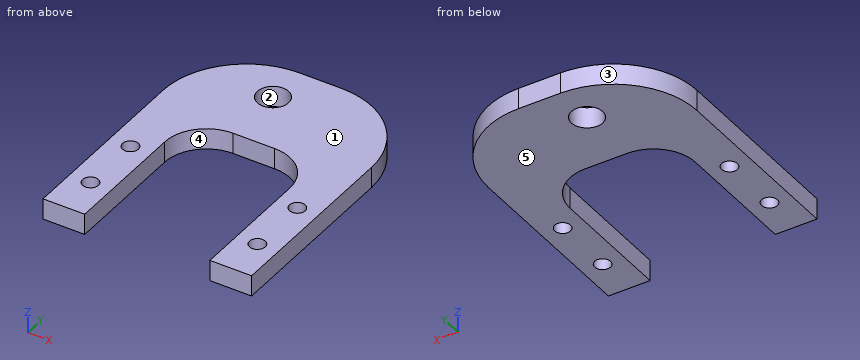
from build123d import *

# Parameters (mm, degrees)
BOSS_EXTRUDE1_DEPTH = 6.35
CUT_EXTRUDE1_REACH  = 8.35
SKETCH2_R           = 2.413
CUT_EXTRUDE2_REACH  = 8.35
SKETCH3_R           = 4.7625
FILLET1_R           = 12.7
FILLET2_R           = 25.4


with BuildPart() as part:
    # Sketch1 → Boss-Extrude1 (new body)
    with BuildSketch(Plane.XY):
        Polygon((0, 0), (12.7, 0), (12.7, 50.8), (50.8, 50.8), (50.8, 0), (63.5, 0), (63.5, 82.55), (0, 82.55), align=None)
    extrude(amount=BOSS_EXTRUDE1_DEPTH)

    # Sketch2 → Cut-Extrude1 (cut, up to next)
    with BuildSketch(Plane.XY.offset(6.35), mode=Mode.PRIVATE) as cut_extrude1_sk1:
        with Locations((6.35, 12.7)):
            Circle(SKETCH2_R)
    cut_extrude1_tool1 = extrude(cut_extrude1_sk1.sketch, amount=-CUT_EXTRUDE1_REACH, mode=Mode.PRIVATE) & part.part
    add(cut_extrude1_tool1.solids().sort_by_distance((6.35, 12.7, 6.35))[0], mode=Mode.SUBTRACT)
    # Sketch2 → Cut-Extrude1 (cut, up to next)
    with BuildSketch(Plane.XY.offset(6.35), mode=Mode.PRIVATE) as cut_extrude1_sk2:
        with Locations((6.35, 31.75)):
            Circle(SKETCH2_R)
    cut_extrude1_tool2 = extrude(cut_extrude1_sk2.sketch, amount=-CUT_EXTRUDE1_REACH, mode=Mode.PRIVATE) & part.part
    add(cut_extrude1_tool2.solids().sort_by_distance((6.35, 31.75, 6.35))[0], mode=Mode.SUBTRACT)
    # Sketch2 → Cut-Extrude1 (cut, up to next)
    with BuildSketch(Plane.XY.offset(6.35), mode=Mode.PRIVATE) as cut_extrude1_sk3:
        with Locations((57.15, 12.7)):
            Circle(SKETCH2_R)
    cut_extrude1_tool3 = extrude(cut_extrude1_sk3.sketch, amount=-CUT_EXTRUDE1_REACH, mode=Mode.PRIVATE) & part.part
    add(cut_extrude1_tool3.solids().sort_by_distance((57.15, 12.7, 6.35))[0], mode=Mode.SUBTRACT)
    # Sketch2 → Cut-Extrude1 (cut, up to next)
    with BuildSketch(Plane.XY.offset(6.35), mode=Mode.PRIVATE) as cut_extrude1_sk4:
        with Locations((57.15, 31.75)):
            Circle(SKETCH2_R)
    cut_extrude1_tool4 = extrude(cut_extrude1_sk4.sketch, amount=-CUT_EXTRUDE1_REACH, mode=Mode.PRIVATE) & part.part
    add(cut_extrude1_tool4.solids().sort_by_distance((57.15, 31.75, 6.35))[0], mode=Mode.SUBTRACT)

    # Sketch3 → Cut-Extrude2 (cut, up to next)
    with BuildSketch(Plane.XY.offset(6.35), mode=Mode.PRIVATE) as cut_extrude2_sk1:
        with Locations((25.4, 69.85)):
            Circle(SKETCH3_R)
    cut_extrude2_tool1 = extrude(cut_extrude2_sk1.sketch, amount=-CUT_EXTRUDE2_REACH, mode=Mode.PRIVATE) & part.part
    add(cut_extrude2_tool1.solids().sort_by_distance((25.4, 69.85, 6.35))[0], mode=Mode.SUBTRACT)

    # Fillet1
    fillet1_edges = [part.edges().sort_by_distance(p)[0] for p in [
        (50.8, 50.8, 3.175),
        (12.7, 50.8, 3.175),
    ]]
    fillet(fillet1_edges, radius=FILLET1_R)

    # Fillet2
    fillet2_edges = [part.edges().sort_by_distance(p)[0] for p in [
        (0, 82.55, 3.175),
        (63.5, 82.55, 3.175),
    ]]
    fillet(fillet2_edges, radius=FILLET2_R)


solid = part.part
Could you check a few things on this model? Use its own coordinates, in mm. Face numbers are marked on the shaded views. A direction names the side the tool comes from. Give positions to 0.01 mm unless a question says otherwise; leave off trailing zeros. Write each loop counter-clockwise with the first axis right and the second up, starting at its lowest first coordinate (ties: lowest second). Pieces come first, ordered by that corner, then holes. Notation, with made-up numbers: (54.25, -17) -> (110.25, -17) arc R7 ccw to (110.25, -12) -> close; hole circle Ø5 at (-16, 51.5). An arc over 180 degrees is marked (long way). Write each question's results on one line, items separated by ' | '. Start each with the question number.
Q1. We'd pull the mould along X, two halves only. Please class the marked faces 1, 2 and 3: +X half, -X half, draft (parallel to the pull), parting line (faces both ways), or undercut.
Q2. I need wall thicknesses on probe 1 along X at (y, z) = (18.5, 1.25); probe 2 along X at (y, z) = (14, 0.5); probe 3 along Y at (x, z) = (6.35, 2). Which ranges of each line are inside material? Lowest first, please.
Q3. Suppose I cut it at B-B, the plane x = 6.35. List the corners of the cut face in (y, z) for me, and give its area (3 significant figures).
Q4. Suppose I cut it at C-C, the plane z = 5.5. State how many separate pieces and enclosed holes the cut face has, and give its area (3 significant figures).
Q5. Suppose I cut it at A-A, the plane y = 31.75. List the corners of the cut face in (x, z) for me.
Q6. Which directions (+Z, -Z, +X, -X, +Y, -Y) give clear straight access to the entire face, cutting with the end or side of a thin tool? Please do the marked faces 4 and 5.
Q7. Suppose I cut it at D-D, the plane y = 69.85. List the corners of the cut face in (x, z) for me.
Outcome:
1) face 1: draft | face 2: undercut | face 3: -X half
2) probe 1: 0 to 12.7, 50.8 to 63.5 | probe 2: 0 to 4.32, 8.38 to 12.7, 50.8 to 55.12, 59.18 to 63.5 | probe 3: 0 to 10.29, 15.11 to 29.34, 34.16 to 73.95
3) outline: (0, 0) -> (10.29, 0) -> (10.29, 6.35) -> (0, 6.35) -> close; (15.11, 0) -> (29.34, 0) -> (29.34, 6.35) -> (15.11, 6.35) -> close; (34.16, 0) -> (73.95, 0) -> (73.95, 6.35) -> (34.16, 6.35) -> close | area: 408 mm2
4) separate pieces: 1 | enclosed holes: 5 | area: 2,950 mm2
5) outline: (0, 0) -> (3.94, 0) -> (3.94, 6.35) -> (0, 6.35) -> close; (8.76, 0) -> (12.7, 0) -> (12.7, 6.35) -> (8.76, 6.35) -> close; (50.8, 0) -> (54.74, 0) -> (54.74, 6.35) -> (50.8, 6.35) -> close; (59.56, 0) -> (63.5, 0) -> (63.5, 6.35) -> (59.56, 6.35) -> close
6) face 4: +Z, -Z, -Y | face 5: -Z, +X, -X, +Y, -Y
7) outline: (3.4, 0) -> (20.64, 0) -> (20.64, 6.35) -> (3.4, 6.35) -> close; (30.16, 0) -> (60.1, 0) -> (60.1, 6.35) -> (30.16, 6.35) -> close
